The model under review builds one solid part; all positions refer to its coordinate system, in mm. A direction names the side the tool comes from. Round coordinates to 2 decimals unless told otherwise and drop trailing zeros. Write each loop counter-clockwise with the first axis right and the second up, starting at its lowest first coordinate (ties: lowest second). Pieces come first, ordered by that corner, then holes. Notation, with made-up numbers: M -38.75,-18.75 L -20.75,-18.75 A13 cw -20.75,-6.75 Z; hole C 68,49 d1. An arc over 180 degrees is marked long. One line per item, written item: value. Start each with the question number.
1) Take a section at A-A, the plane y = 45. Write out the cut boundary in (x, z).
2) Wall thickness on probe 1 along Y at (x, z) = (-50, 1.75); probe 2 along Y at (x, z) = (-46.5, 4.05); probe 3 along Y at (x, z) = (-78, 3.9): over which ranges is each line inside the solid? List them lowest first.
3) For P1, Ø5, axis at x = -59.5, y = 53, coming from the -Z side; P2, Ø1.5, axis at y = 56.5, z = 0.5, coming from the -X side; P3, Ø2.5, axis at x = -37.5, z = 2.5, coming from the -Y side, all flat-tipped, find the tip position at first contact; note any pin that passes through.
4) Take a section at C-C, the plane z = 3.7. Write out the cut boundary in (x, y), and give its area (3 significant figures).
5) Mouldability with a two-part tool opening along Y and no side actions: class faces 1 (the face through (-54, 20, 2)), 2 (the face through (-69, 46, 0)), 3 (the face through (-89.97, 43.47, 2.46)) as +Y half, -Y half, draft (parallel to the pull), parting line (faces both ways), or undercut.
6) Take a section at D-D, the plane y = 56.5. Write out the cut boundary in (x, z).
7) Tool access review of faces 4 (the face through (-54, 70, 2)), 5 (the face through (-31, 29.001, 2)): name each direction out of +Z, -Z, +X, -X, +Y, -Y from which nothing blocks a thin tool from reaching the whole face with its end or side.
8) Take a section at B-B, the plane x = -43.5. Write out the cut boundary in (y, z).
Autodesk Fusion 360 part; units mm, degrees
sketch "Sketch1" plane through (0, 0, 0) normal (0, 0, 1) x (1, 0, 0)
  circle A0 centre (-50, 73) radius 5
  circle A1 centre (-50, 17) radius 5
  circle A2 centre (-78, 45) radius 5
  line L0 (-50.0531, 60.9999) -> (-49.9469, 60.9999)
  line L1 (-50.1491, 29.0007) -> (-49.8509, 29.0007)
  arc A3 (-49.9469, 60.9999) -> (-49.8509, 29.0007) centre (-50, 45) ccw
  line L2 (-50.0531, 60.9999) -> (-13.3394, 60.9999)
  line L3 (-13.3391, 29.0007) -> (-50.1491, 29.0007)
  arc A4 (-13.3394, 60.9999) -> (-13.3391, 29.0007) centre (-50, 45) ccw
  dimension "d1" = 80
  dimension "d3" = 10
  dimension "d5" = 10
  dimension "d7" = 10
extrude "Extrude1" add sketch "Sketch1" along normal blind 5
Checked values:
1. outline: M -90,0 L -83,0 L -83,5 L -90,5 Z; M -73,0 L -66,0 L -66,5 L -73,5 Z
2. probe 1: y = 5 to 12, 22 to 29, 61 to 68, 78 to 85
2. probe 2: y = 5.15 to 13.43, 20.57 to 29, 61 to 69.43, 76.57 to 84.85
2. probe 3: y = 16.43 to 40, 50 to 73.57
3. P1: passes through
3. P2: stops at x = -88.53
3. P3: stops at y = 6.61
4. outline: M -50.15,29 A16 cw -50.05,61 L -13.34,61 A40 ccw long -13.34,29 Z; hole C -78,45 d10; hole C -50,17 d10; hole C -50,73 d10
4. area: 3,140 mm2
5. face 1: undercut
5. face 2: draft
5. face 3: parting line
6. outline: M -88.31,0 L -61.12,0 L -61.12,5 L -88.31,5 Z
7. face 4: +Z, -Z
7. face 5: +Z, -Z, +X
8. outline: M 5.53,0 L 29,0 L 29,5 L 5.53,5 Z; M 61,0 L 84.47,0 L 84.47,5 L 61,5 Z
